Design review of the part built by this model. Coordinates are the model's own, in mm. Face numbers are marked on the shaded views. Coordinates: 2 decimals unless noted, no trailing zeros. Write each loop counter-clockwise with the first axis right and the second up, starting at its lowest first coordinate (ties: lowest second). Pieces come first, ordered by that corner, then holes.
Q1. For pin 1 Ø7 at (x, y) = (90, -25) entering from +Z; pin 2 Ø0.5 at (x, z) = (21, 3.5) entering from +Y; pin 3 Ø1.6 at (x, z) = (31, 1) entering from +Y; pin 4 Ø3.5 at (x, y) = (37, -1.5) entering from -Z, all flat-tipped, find the tip position at first contact; note any pin that passes through.
Q2. Take a section at A-A, the plane y = -25. Write out the cut boundary in (x, z), plus the area to 3 significant figures.
Q3. For L1, parallel to X at y = -25, z = 2.75; L2, parallel to Y at x = 28.5, z = 3.2; L3, parallel to Y at x = 90, z = 0.8, list the stretches that pass through material, from the lowest coordinate up.
Q4. The part is to be moulded in two halves that separate along Y. For the marked faces 1 and 2, say which applies: released by +Y, released by -Y, zero draft, split by the parting line, or undercut.
Q5. Take a section at D-D, the plane y = -38.5. Write out the cut boundary in (x, z).
Q6. Take a section at C-C, the plane x = 73. Write out the cut boundary in (y, z).
Q7. Take a section at B-B, the plane x = 90. Write out the cut boundary in (y, z).
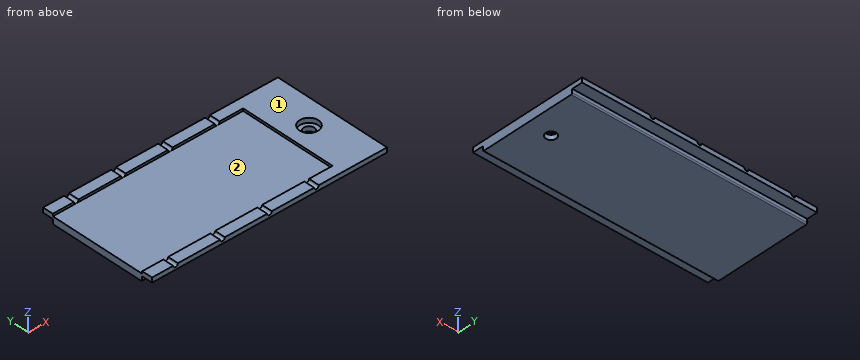
Autodesk Inventor part; units mm, degrees
ref_plane "YZ Plane" through (0, 0, 0) normal (1, 0, 0) x (0, 1, 0)
ref_plane "XZ Plane" through (0, 0, 0) normal (0, 1, 0) x (-1, 0, 0)
ref_plane "XY Plane" through (0, 0, 0) normal (0, 0, 1) x (1, 0, 0)
sketch "Sketch1" plane through (0, 0, 0) normal (0, 0, 1) x (1, 0, 0)
  line L0 (0, 0) -> (100, 0)
  line L1 (100, 0) -> (100, -50)
  line L2 (100, -50) -> (0, -50)
  line L3 (0, -50) -> (0, 0)
  dimension "d2" = 100
  dimension "d3" = 50
extrude "Extrusion1" add sketch "Sketch1" along normal blind 4
sketch "Sketch2" plane through (0, 0, 0) normal (0, 0, -1) x (-1, 0, 0)
  line L0 (0, 0) -> (0, -50)
  line L1 (0, -50) -> (-100, -50)
  line L2 (-100, -50) -> (-100, -45.5)
  line L3 (-100, -45.5) -> (0, -45.5)
  line L4 (0, -45.5) -> (0, -50)
  line L5 (0, 0) -> (-100, 0)
  line L6 (-100, 0) -> (-100, -4.5)
  line L7 (-100, -4.5) -> (0, -4.5)
  line L8 (0, -4.5) -> (0, 0)
  line L9 (-100, -50) -> (-100, 0)
  dimension "d6" = 4.5
  dimension "d7" = 4.5
  dimension "d16" = 0
  dimension "d17" = 0
extrude "Extrusion2" cut sketch "Sketch2" against normal blind 2 contours L0 L7 L6 L5 | L0 L1 L2 L3
fillet "Fillet1" radius 0.5 2 edges at (50, -45.5, 0) (50, -4.5, 0)
sketch "Sketch3" plane through (0, 0, 4) normal (0, 0, 1) x (1, 0, 0)
  line L0 (0, -45) -> (0, -5)
  line L1 (0, -4.5) -> (81, -4.5)
  line L2 (81, -4.5) -> (81, -45.5)
  line L3 (81, -45.5) -> (0, -45.5)
  line L4 (0, -45.5) -> (0, -4.5)
  line L5 (100, 0) -> (0, 0)
  dimension "d11" = 81
  dimension "d12" = 41
  dimension "d13" = 4.5
extrude "Extrusion3" cut sketch "Sketch3" against normal blind 1
sketch "Sketch5" plane through (0, 0, 4) normal (0, 0, 1) x (1, 0, 0)
  line L0 (100, 0) -> (0, 0)
  line L1 (100, -50) -> (100, 0)
  point P0 (90, -25)
  dimension "d37" = 25
  dimension "d38" = 10
hole "Hole1" at (90, -25, 4) direction (0, 0, -1) diameter 4.5 end through all counterbore diameter 8 counterbore depth 2
hole "Hole2" at (10, -50, 4) direction (0, 1, 0) diameter 2 end through all
pattern_linear "Rectangular Pattern1" count 4 spacing 20 along (1, 0, 0) of "Hole2"
properties part number "TNS_Greiferbacke_MA_Jun_T2"
Responses:
1. pin 1: stops at z = 2
1. pin 2: stops at y = 0
1. pin 3: stops at y = -4.5
1. pin 4: stops at z = 2
2. outline: (0, 0) - (87.75, 0) - (87.75, 2) - (86, 2) - (86, 4) - (81, 4) - (81, 3) - (0, 3) - close; (92.25, 0) - (100, 0) - (100, 4) - (94, 4) - (94, 2) - (92.25, 2) - close
2. area: 294 mm2
3. L1: x = 0 to 86, 94 to 100
3. L2: y = -50 to -45.5, -4.5 to 0
3. L3: y = -45.5 to -27.25, -22.75 to -4.5
4. face 1: zero draft
4. face 2: undercut
5. outline: (0, 0) - (100, 0) - (100, 4) - (81, 4) - (81, 3) - (0, 3) - close
6. outline: (-50, 2) - (-45.5, 2) - (-45.5, 0.5) arc R0.5 ccw to (-45, 0) - (-5, 0) arc R0.5 ccw to (-4.5, 0.5) - (-4.5, 2) - (0, 2) - (0, 4) - (-4.5, 4) - (-4.5, 3) - (-45.5, 3) - (-45.5, 4) - (-50, 4) - close
7. outline: (-50, 2) - (-45.5, 2) - (-45.5, 0.5) arc R0.5 ccw to (-45, 0) - (-27.25, 0) - (-27.25, 2) - (-29, 2) - (-29, 4) - (-50, 4) - close; (-22.75, 0) - (-5, 0) arc R0.5 ccw to (-4.5, 0.5) - (-4.5, 2) - (0, 2) - (0, 4) - (-21, 4) - (-21, 2) - (-22.75, 2) - close
